Source: CAD feature listing. Evaluate the final solid. Frame: model axes, mm. A direction names the side the tool comes from. Round coordinates to 2 decimals unless told otherwise and drop trailing zeros. Write each loop counter-clockwise with the first axis right and the second up, starting at its lowest first coordinate (ties: lowest second). Pieces come first, ordered by that corner, then holes. Notation, with made-up numbers: M 25,9 L 34,9 A12 ccw 34,29 Z; hole C 32.25,86.5 d9. An arc over 180 degrees is marked long. Use a Markdown table: item, result.
```python
from build123d import *

# Parameters (mm, degrees)
SKETCH1_R           = 4
BOSS_EXTRUDE1_DEPTH = 10
SKETCH2_W           = 18
SKETCH2_H           = 5
SKETCH2_W_2         = 5
SKETCH2_H_2         = 18
BOSS_EXTRUDE2_DEPTH = 15


with BuildPart() as part:
    # Sketch1 → Boss-Extrude1 (new body)
    with BuildSketch(Plane.XY):
        Polygon((11.202614379, -118.751633987), (177.202614379, -118.751633987), (177.202614379, -100.751633987), (11.202614379, -100.751633987), (11.202614379, 9.248366013), (-6.797385621, 9.248366013), (-6.797385621, -228.751633987), (11.202614379, -228.751633987), align=None)
        with Locations((2.202614379, -109.751633987)):
            Circle(SKETCH1_R, mode=Mode.SUBTRACT)
    extrude(amount=BOSS_EXTRUDE1_DEPTH)

    # Sketch2 → Boss-Extrude2 (add)
    with BuildSketch(Plane(origin=(0, 0, 0), x_dir=(-1, 0, 0), z_dir=(0, 0, -1))):
        with Locations((-2.202614379, -231.251633987)):
            Rectangle(SKETCH2_W, SKETCH2_H)
        with Locations((-179.702614379, -109.751633987)):
            Rectangle(SKETCH2_W_2, SKETCH2_H_2)
        with Locations((-2.202614379, 11.748366013)):
            Rectangle(SKETCH2_W, SKETCH2_H)
    extrude(amount=-BOSS_EXTRUDE2_DEPTH)


solid = part.part
```
Q1. Mould query, pull axis Y, two halves, no side actions, for faces 1 (the flat face through (-6.797, -111, 4)), 2 (the flat face through (37, -109, 10)), 3 (the flat face through (98, -100.752, 4)). Classes: +Y half, -Y half, draft (parallel to the pull), parting line (faces both ways), or undercut.
Results are:
| item | result |
|---|---|
| face 1 | draft |
| face 2 | undercut |
| face 3 | +Y half |
Q2. Reachability of faces 4 (the flat face through (2, -231, 15)), 5 (the flat face through (96, -118.752, 4)), 6 (the flat face through (2, 9.248, 12)), 7 (the flat face through (11.203, -44, 4)), 8 (the flat face through (177.203, -110, 12)) from +Z, -Z, +X, -X, +Y, -Y: full face, straight path, thin tool, end or side. Return the list, or none.
Results are:
| item | result |
|---|---|
| face 4 | +Z, +X, -X, +Y, -Y |
| face 5 | +Z, -Z, +X, -Y |
| face 6 | +Z, +X, -X |
| face 7 | +Z, -Z, +X, +Y |
| face 8 | +Z, -X, +Y, -Y |
Q3. Section A-A on z = 7.75. Return loops of the section in (x, y).
Results are:
| item | result |
|---|---|
| outline | M -6.8,-233.75 L 11.2,-233.75 L 11.2,-118.75 L 182.2,-118.75 L 182.2,-100.75 L 11.2,-100.75 L 11.2,14.25 L -6.8,14.25 Z; hole C 2.2,-109.75 d8 |
Q4. First-contact query: pin 1 Ø4 at (x, z) = (21.5, 6) entering from -Y; pin 2 Ø6 at (x, z) = (139.5, 5) entering from +Y; pin 3 Ø5.5 at (y, z) = (-106.5, 13) entering from -X; pin 4 Ø5 at (y, z) = (-11, 11) entering from -X. Flat tips, straight axial feed; report the tip coordinate or a pass-through.
Results are:
| item | result |
|---|---|
| pin 1 | y = -118.75 |
| pin 2 | y = -100.75 |
| pin 3 | x = 177.2 |
| pin 4 | x = -6.8 |
Q5. Line query: L1, parallel to Y at x = 4, z = 12.5; L2, parallel to Y at x = 130, z = 4.25; L3, parallel to X at y = -44.5, z = 6.25. Output: solid intervals per line, ascending.
Results are:
| item | result |
|---|---|
| L1 | -233.75 to -228.75, 9.25 to 14.25 |
| L2 | -118.75 to -100.75 |
| L3 | -6.8 to 11.2 |
Q6. Section B-B on y = -17.5. Return loops of the section in (x, z).
Results are:
| item | result |
|---|---|
| outline | M -6.8,0 L 11.2,0 L 11.2,10 L -6.8,10 Z |
Q7. Section C-C on x = 121.5. Return loops of the section in (y, z).
Results are:
| item | result |
|---|---|
| outline | M -118.75,0 L -100.75,0 L -100.75,10 L -118.75,10 Z |
